Autodesk Inventor part; units mm, degrees
ref_plane "YZ Plane" through (0, 0, 0) normal (1, 0, 0) x (0, 1, 0)
ref_plane "XZ Plane" through (0, 0, 0) normal (0, 1, 0) x (-1, 0, 0)
ref_plane "XY Plane" through (0, 0, 0) normal (0, 0, 1) x (1, 0, 0)
sketch "Sketch2" plane through (0, 0, 0) normal (1, 0, 0) x (0, 1, 0)
  line L0 (0, 0) -> (14, 0)
  line L1 (14, 0) -> (14, -32)
  line L2 (14, -32) -> (0, -32) construction
  line L3 (0, -32) -> (0, 0)
  circle A0 centre (7, -25) radius 1.5
  line L4 (14, -32) -> (14, -52)
  line L5 (14, -52) -> (0, -52)
  line L6 (0, -52) -> (0, -32)
  line L7 (7, -19.5) -> (7, -30.5) construction
  line L8 (5.5, -19.5) -> (5.5, -30.5)
  line L9 (8.5, -30.5) -> (8.5, -19.5)
  arc A1 (8.5, -19.5) -> (5.5, -19.5) centre (7, -19.5) ccw
  arc A2 (5.5, -30.5) -> (8.5, -30.5) centre (7, -30.5) ccw
  point P0 (7, -32)
  dimension "d5" = 32
  dimension "d6" = 14
  dimension "d7" = 3
  dimension "d8" = 7
  dimension "d11" = 20
extrude "Extrusion1" add sketch "Sketch2" along normal blind 3
sketch "Sketch3" plane through (3, 0, 0) normal (1, 0, 0) x (0, 0, -1)
  line L0 (52, 14) -> (42, 14)
  line L1 (42, 14) -> (42, 9)
  line L2 (42, 9) -> (52, 9)
  line L3 (52, 9) -> (52, 14)
  line L4 (52, 0) -> (52, 14)
  line L5 (52, 14) -> (0, 14)
  dimension "d12" = 5
  dimension "d13" = 10
extrude "Extrusion2" add sketch "Sketch3" along normal blind 10
sketch "Sketch4" plane through (3, 9, -42) normal (0, -1, 0) x (1, 0, 0)
  circle A0 centre (5, -5) radius 1.5
  line L0 (10, 0) -> (10, -10)
  point P0 (-3, 42)
  point P1 (10, -5)
  dimension "d16" = 3
  dimension "d17" = 5
extrude "Extrusion3" cut sketch "Sketch4" against normal through all
properties part number "IRSensorMount"
Geometry check sheet. Reference: the model listing, model coordinates, mm. A direction names the side the tool comes from. Give positions to 0.01 mm unless a question says otherwise; leave off trailing zeros. Write each loop counter-clockwise with the first axis right and the second up, starting at its lowest first coordinate (ties: lowest second). Pieces come first, ordered by that corner, then holes. Notation, with made-up numbers: M -30,-15.75 L 17,-15.75 A26 cw 17,14.25 Z; hole C 73,-8.75 d10. An arc over 180 degrees is marked long. Answer as CSV lines item,"result". Start each with the question number.
Q1. Go/stop test with flat-tipped pins: pin 1 (2 mm diameter, centred on y = 12.5, z = -33.5, fed in from +X); pin 2 (6 mm diameter, centred on x = 7.5, z = -46.5, fed in from -Y); pin 3 (5.5 mm diameter, centred on x = 9.5, y = 12.5, fed in from +Z). Record where each tip stops, or that it passes through.
Q2. Section check C-C, the plane z = -47. Record the cut outline in (x, y).
Q3. Material ranges on L1, parallel to Z at x = 8, y = 10.8; L2, parallel to Y at x = 4.25, z = -46; L3, parallel to X at y = 13.5, z = -32, recorded low to high.
Q4. Section check D-D, the plane x = 8. Record the cut outline in (y, z), then the cut area to 3 significant figures.
Q5. Section check B-B, the plane x = 1.5. Record the cut outline in (y, z), then the cut area to 3 significant figures.
Q6. Section check A-A, the plane y = 13. Record the cut outline in (x, z), then the cut area to 3 significant figures.
Q7. Release check for a two-part mould opening along Z. For faces 1 (the face through (6.8, 9, -45.8)), 2 (the face through (8, 12, -42)), 3 (the face through (1, 5.5, -25)) record: pulls with the +Z half, pulls with the -Z half, needs draft (parallel to the pull), parting line crosses it, or undercut.
Q8. Tool access check on faces 4 (the face through (2, 14, -37)), 5 (the face through (1, 7, -18)). Record the directions out of +Z, -Z, +X, -X, +Y, -Y that give a thin tool (end or side, any length) a straight path to the whole face; none if there is none.
Geometry says:
1,pin 1,"x = 3"
1,pin 2,"y = 9"
1,pin 3,"z = -42"
2,outline,"M 0,0 L 3,0 L 3,9 L 6.5,9 L 6.5,14 L 0,14 Z; M 9.5,9 L 13,9 L 13,14 L 9.5,14 Z"
3,L1,"-52 to -48.5, -45.5 to -42"
3,L2,"9 to 14"
3,L3,"0 to 3"
4,outline,"M 9,-52 L 14,-52 L 14,-48.5 L 9,-48.5 Z; M 9,-45.5 L 14,-45.5 L 14,-42 L 9,-42 Z"
4,area,"35.0 mm^2"
5,outline,"M 0,-52 L 14,-52 L 14,0 L 0,0 Z; hole M 5.5,-30.5 A1.5 ccw 8.5,-30.5 L 8.5,-19.5 A1.5 ccw 5.5,-19.5 Z"
5,area,"688 mm^2"
6,outline,"M 0,-52 L 13,-52 L 13,-42 L 3,-42 L 3,0 L 0,0 Z; hole C 8,-47 d3"
6,area,"249 mm^2"
7,face 1,"needs draft"
7,face 2,"pulls with the +Z half"
7,face 3,"undercut"
8,face 4,"+Z, -Z, +X, -X, +Y"
8,face 5,"+X, -X"
